Here's the drawing with two shaded views (mm, measured from the low corner). I have some questions. A direction names the side the tool comes from. Round coordinates to 2 decimals unless told otherwise and drop trailing zeros. Order: outer loops, then holes, each group sorted by start corner. A loop starts at its lowest first (then second) coordinate and runs counter-clockwise, first axis right, second up. Notation, with made-up numbers: (42.5, 52) - (87.5, 52) arc R24 ccw to (87.5, 81) - close; hole circle Ø9 at (-14, -20). An arc over 180 degrees is marked (long way). One line per item, written item: value.
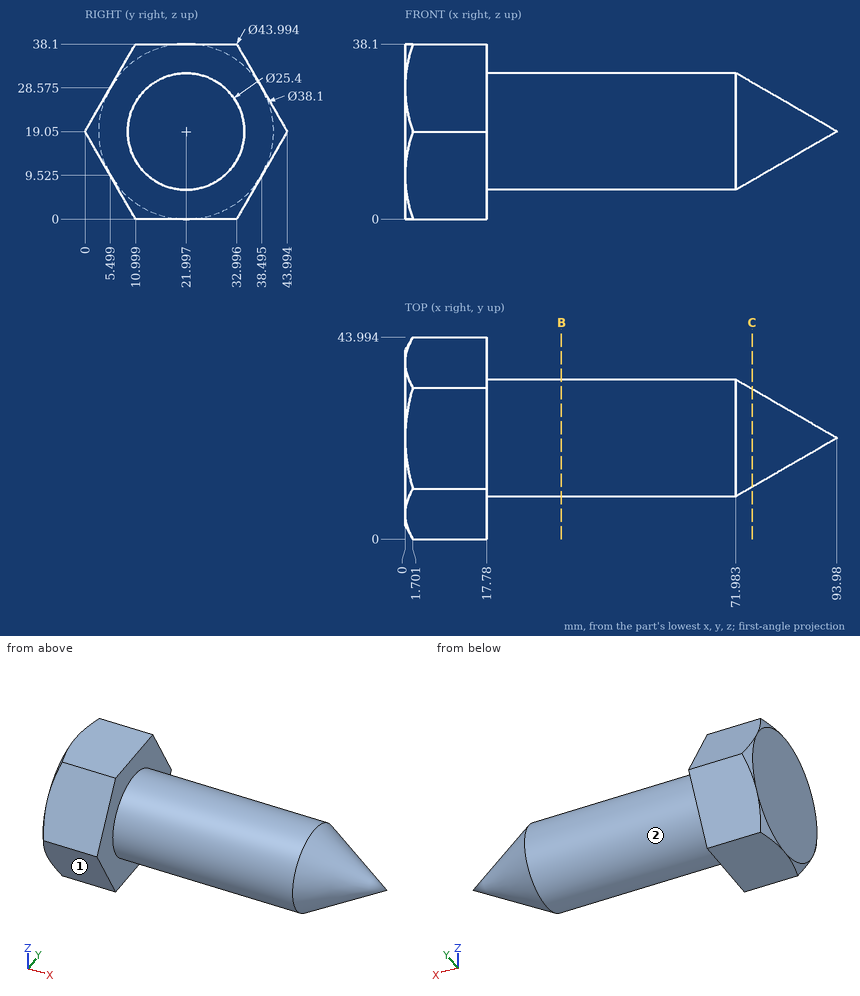
Q1. If we section it at C-C, the plane x = 75.5: Please give me the cut outline in (y, z).
Results list:
outline: circle Ø21.34 at (22, 19.05)
Q2. Will these pins go through, and if not, where does the flat tip stop? pin 1 (3 mm diameter, centred on y = 12, z = 28, fed in from +X) (1 decimal); pin 2 (1 mm diameter, centred on y = 25, z = 14, fed in from +X); pin 3 (3 mm diameter, centred on x = 14.5, z = 29, fed in from +Y) (1 decimal).
Results list:
pin 1: x = 73.3
pin 2: x = 84.67
pin 3: y = 39.1
Q3. If we section it at B-B, the plane x = 34: Please give me the cut outline in (y, z).
Results list:
outline: circle Ø25.4 at (22, 19.05)
Q4. Which directions (+Z, -Z, +X, -X, +Y, -Y) give clear straight access to the entire face, cutting with the end or side of a thin tool? Please do the marked faces 1 and 2.
Results list:
face 1: -Z, +X, -X, -Y
face 2: +X
Q5. If I drill on line 1 along X through (y, z) = (26.5, 3); line 2 along X through (y, z) = (14, 28); line 3 along Y through (x, z) = (44.5, 17.5), over which ranges is the centre line in solid material (lowest first)?
Results list:
line 1: 0 to 17.78
line 2: 0 to 73.19
line 3: 9.39 to 34.6
